from build123d import *

# Parameters (mm, degrees)
F0_R     = 23
F1_DEPTH = 4
F2_R     = 23
F2_R_2   = 21
F3_DEPTH = 4
F4_R     = 6.5
F5_DEPTH = 4


with BuildPart() as f1:
    # F0 (on Top) → F1 (new body)
    with BuildSketch(Plane.XY):
        Circle(F0_R)
    extrude(amount=F1_DEPTH)

    # F2 (on face) → F3 (join)
    with BuildSketch(Plane.XY.offset(4)):
        Circle(F2_R)
        Circle(F2_R_2, mode=Mode.SUBTRACT)
    extrude(amount=F3_DEPTH)

    # F4 (on face) → F5 (cut, through all)
    with BuildSketch(Plane.XY.offset(4)):
        Circle(F4_R)
    extrude(amount=-F5_DEPTH, mode=Mode.SUBTRACT)


solid = f1.part
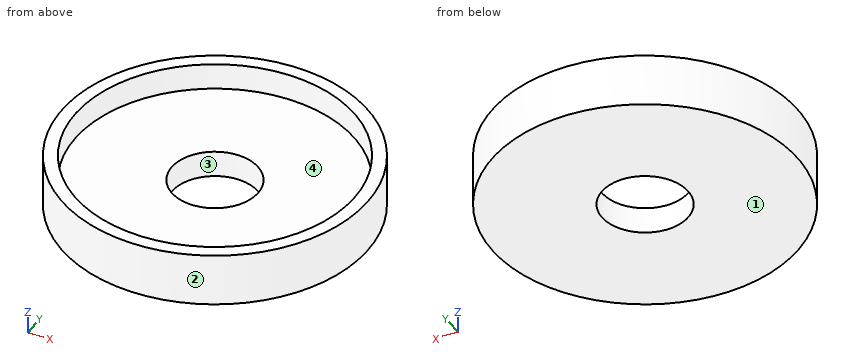
CAD build for the part. Positions are in the model's coordinates, mm. Face numbers are marked on the shaded views. Give positions to 0.01 mm unless a question says otherwise; leave off trailing zeros. Order: outer loops, then holes, each group sorted by start corner. A loop starts at its lowest first (then second) coordinate and runs counter-clockwise, first axis right, second up. Notation, with made-up numbers: (60.5, -31.75) - (86.5, -31.75) arc R24 ccw to (86.5, -13.75) - close; hole circle Ø9 at (43.25, -29.5). An arc over 180 degrees is marked (long way). Answer in a Markdown table with one row per item.
1. Saw through at C-C, the plane z = 1.75. Give the cut face in (x, y), plus the area to 3 significant figures.
Data:
| item | result |
|---|---|
| outline | circle Ø46 at (0, 0); hole circle Ø13 at (0, 0) |
| area | 1,530 mm² |
2. Saw through at D-D, the plane x = -11. Give the cut face in (y, z).
Data:
| item | result |
|---|---|
| outline | (-20.2, 0) - (20.2, 0) - (20.2, 8) - (17.89, 8) - (17.89, 4) - (-17.89, 4) - (-17.89, 8) - (-20.2, 8) - close |
3. Saw through at A-A, the plane x = 0. Give the cut face in (y, z), plus the area to 3 significant figures.
Data:
| item | result |
|---|---|
| outline | (-23, 0) - (-6.5, 0) - (-6.5, 4) - (-21, 4) - (-21, 8) - (-23, 8) - close; (6.5, 0) - (23, 0) - (23, 8) - (21, 8) - (21, 4) - (6.5, 4) - close |
| area | 148 mm² |
4. Probe probe 1 along Y at (x, z) = (0, 3.1); probe 2 along Y at (x, z) = (0, 5.85); probe 3 along Z at (x, y) = (15, 11). List the from-to ranges inside material, lowest first. Write a range as [from, to].
Data:
| item | result |
|---|---|
| probe 1 | y = [-23, -6.5], [6.5, 23] |
| probe 2 | y = [-23, -21], [21, 23] |
| probe 3 | z = [0, 4] |
5. Pull direction X, two halves, no side cores. Call the marked faces 1, 2, 3 and 4: pulls with the +X half, pulls with the -X half, needs draft (parallel to the pull), parting line crosses it, or undercut.
Data:
| item | result |
|---|---|
| face 1 | needs draft |
| face 2 | parting line crosses it |
| face 3 | undercut |
| face 4 | undercut |
6. Flat gauge pins, fed straight in: pin 1 (1.5 mm diameter, centred on y = 1.5, z = 4, fed in from +X); pin 2 (1 mm diameter, centred on x = 13, y = -17, fed in from -Z); pin 3 (12 mm diameter, centred on x = 3.5, y = 10.5, fed in from +Z); pin 4 (4 mm diameter, centred on y = -3, z = 3.5, fed in from -X). Where does each tip first touch, or does it go through?
Data:
| item | result |
|---|---|
| pin 1 | stops at x = 22.99 |
| pin 2 | stops at z = 0 |
| pin 3 | stops at z = 4 |
| pin 4 | stops at x = -22.98 |
